CAD build for the part. Positions are in the model's coordinates, mm. A direction names the side the tool comes from. Coordinates: 2 decimals unless noted, no trailing zeros. Order: outer loops, then holes, each group sorted by start corner. A loop starts at its lowest first (then second) coordinate and runs counter-clockwise, first axis right, second up. Notation, with made-up numbers: M -0.5,55.25 L 38.5,55.25 A5 cw 38.5,62.25 Z; hole C -29,30.5 d9. An arc over 180 degrees is marked long. One line per item, written item: value.
from build123d import *

# Parameters (mm, degrees)
SKETCH1_W                = 30.1752
SKETCH1_H                = 12.7
BOSS_EXTRUDE1_DEPTH      = 6.35
BOSS_EXTRUDE1_DEPTH_BACK = 6.35
SKETCH2_W                = 17.4752
SKETCH2_H                = 6.6675
CUT_EXTRUDE1_DEPTH       = 6.35
CUT_EXTRUDE1_DEPTH_BACK  = 6.35
HOLE1_D                  = 6.79196
HOLE1_DEPTH              = 11.176
HOLE1_CSINK_D            = 7.9375
HOLE1_CSINK_ANGLE        = 90
HOLE2_D                  = 6.79196
HOLE2_DEPTH              = 1.524


with BuildPart() as part:
    # Sketch1 → Boss-Extrude1 (new body, two sides)
    with BuildSketch(Plane.XY) as boss_extrude1_sk:
        with Locations((8.7376, 0)):
            Rectangle(SKETCH1_W, SKETCH1_H)
    extrude(amount=BOSS_EXTRUDE1_DEPTH)
    extrude(boss_extrude1_sk.sketch, amount=-BOSS_EXTRUDE1_DEPTH_BACK)

    # Sketch2 → Cut-Extrude1 (cut, two sides)
    with BuildSketch(Plane(origin=(0, 0, 0), x_dir=(1, 0, 0), z_dir=(0, 1, 0))) as cut_extrude1_sk:
        with Locations((2.3876, 0)):
            Rectangle(SKETCH2_W, SKETCH2_H)
    extrude(amount=CUT_EXTRUDE1_DEPTH, mode=Mode.SUBTRACT)
    extrude(cut_extrude1_sk.sketch, amount=-CUT_EXTRUDE1_DEPTH_BACK, mode=Mode.SUBTRACT)

    # Hole1
    with Locations(Plane(origin=(23.8252, 0, 0), x_dir=(0, 0, -1), z_dir=(1, 0, 0))):
        with Locations((0, 0)):
            CounterSinkHole(HOLE1_D / 2, HOLE1_CSINK_D / 2, depth=HOLE1_DEPTH, counter_sink_angle=HOLE1_CSINK_ANGLE)

    # Hole2
    with Locations(Plane(origin=(12.6492, 0, 0), x_dir=(0, 0, -1), z_dir=(1, 0, 0))):
        with Locations((0, 0)):
            Hole(HOLE2_D / 2, depth=HOLE2_DEPTH)

    # Sketch7 → Cut-Revolve1 (revolve, cut)
    with BuildSketch(Plane(origin=(0, 0, 0), x_dir=(0, 0, -1), z_dir=(1, 0, 0))):
        Polygon((-6.35, 0), (-6.35, 4.33705), (-5.207, 3.19405), (5.207, 3.19405), (6.35, 4.33705), (6.35, 0), align=None)
    revolve(axis=Axis((0, 0, -6.35), (0, 0, 1)), mode=Mode.SUBTRACT)

    # Sketch8 → Cut-Revolve2 (revolve, cut)
    with BuildSketch(Plane.XY):
        with BuildLine():
            Line((23.8252, 0), (23.8252, 6.35))
            ThreePointArc((23.8252, 6.35), (22.869586956, 9.650754782), (21.2852, 12.7))
            Line((21.2852, 12.7), (30.1752, 12.7))
            Line((30.1752, 12.7), (30.1752, 0))
            Line((30.1752, 0), (23.8252, 0))
        make_face()
    revolve(axis=Axis((30.1752, 0, 0), (-1, 0, 0)), mode=Mode.SUBTRACT)

    # Sketch9 → Cut-Revolve3 (revolve, cut)
    with BuildSketch(Plane.XY):
        with BuildLine():
            Line((-12.7, 0), (-12.7, 12.7))
            Line((-12.7, 12.7), (-3.81, 12.7))
            ThreePointArc((-3.81, 12.7), (-5.394386956, 9.650754782), (-6.35, 6.35))
            Line((-6.35, 6.35), (-6.35, 0))
            Line((-6.35, 0), (-12.7, 0))
        make_face()
    revolve(axis=Axis((-6.35, 0, 0), (-1, 0, 0)), mode=Mode.SUBTRACT)


solid = part.part
Q1. Pin check, flat tips, straight feed: pin 1 Ø7.5 at (x, y) = (0, 0) entering from -Z; pin 2 Ø3 at (y, z) = (-4.5, 0.5) entering from -X. Stop position of each tip, or through.
Recorded:
pin 1: stops at z = -5.76
pin 2: stops at x = 11.13
Q2. Mould opens along Y. For faces 3 (the face through (11.125, 5, 0)), 4 (the face through (12, 6.35, 0)), 5 (the face through (-0.959, 3.047, 4.257)) say: released by +Y, released by -Y, zero draft, split by the parting line, or undercut.
Recorded:
face 3: zero draft
face 4: released by +Y
face 5: undercut
Q3. Which spindle directions (+Z, -Z, +X, -X, +Y, -Y) get a long thin tool onto all of the face, cutting with end or side? Do faces 1 (the face through (11.125, -5, 0)), 2 (the face through (23.825, -3, -3)). Say none if no direction does.
Recorded:
face 1: -X, +Y, -Y
face 2: +Z, -Z, +X, +Y, -Y
Q4. Slice it at D-D (y = -2). Give the number of separate pieces and of enclosed holes in the cut face, plus the area to 3 significant figures.
Recorded:
separate pieces: 4
enclosed holes: 0
area: 163 mm^2
Q5. Slice it at B-B (x = 0). List the corners of the cut face in (y, z).
Recorded:
outline: M -6.35,-6.35 L -4.34,-6.35 L -3.19,-5.21 L -3.19,-3.33 L -6.35,-3.33 Z; M -6.35,3.33 L -3.19,3.33 L -3.19,5.21 L -4.34,6.35 L -6.35,6.35 Z; M 3.19,-5.21 L 4.34,-6.35 L 6.35,-6.35 L 6.35,-3.33 L 3.19,-3.33 Z; M 3.19,3.33 L 6.35,3.33 L 6.35,6.35 L 4.34,6.35 L 3.19,5.21 Z
Q6. Slice it at A-A (x = 10). List the corners of the cut face in (y, z).
Recorded:
outline: M -6.35,-6.35 L 6.35,-6.35 L 6.35,-3.33 L -6.35,-3.33 Z; M -6.35,3.33 L 6.35,3.33 L 6.35,6.35 L -6.35,6.35 Z
Q7. Drill centre lines: line 1 along Y through (x, z) = (0, -4.05); line 2 along Z through (x, y) = (-2, 5.5); line 3 along Z through (x, y) = (19, 0). Where is each one in solid material? Low to high.
Recorded:
line 1: y = -6.35 to -3.19, 3.19 to 6.35
line 2: z = -6.35 to -3.33, 3.33 to 6.35
line 3: z = -6.35 to -3.4, 3.4 to 6.35
Q8. Slice it at C-C (x = 19.5). List the corners of the cut face in (y, z).
Recorded:
outline: M -6.35,-6.35 L 6.35,-6.35 L 6.35,6.35 L -6.35,6.35 Z; hole C 0,0 d6.79
